Source: CAD feature listing. Evaluate the final solid. Frame: model axes, mm. Face numbers are marked on the shaded views. Round coordinates to 2 decimals unless told otherwise and drop trailing zeros. Loops run counter-clockwise (first coordinate to the right, second up) from the corner with the lowest first, then second, coordinate; pieces in that order, holes last. Notation, with made-up numbers: M 13,88.25 L 68,88.25 A24 cw 68,108.25 Z; hole C 29.5,28.5 d1. An arc over 180 degrees is marked long. One line per item, written item: value.
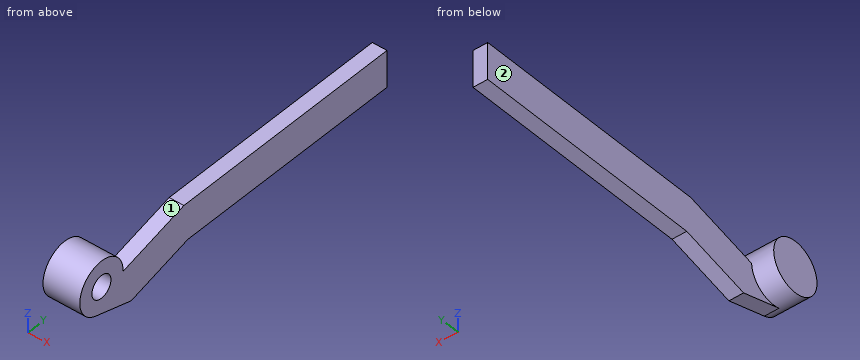
from build123d import *

# Parameters (mm, degrees)
SKETCH1_R           = 7
SKETCH1_R_2         = 3.0845
BOSS_EXTRUDE1_DEPTH = 10
BOSS_EXTRUDE2_START = 7
SKETCH1_3_R         = 7
BOSS_EXTRUDE2_DEPTH = 3
BOSS_EXTRUDE3_DEPTH = 4


with BuildPart() as part:
    # Sketch1 → Boss-Extrude1 (new body)
    with BuildSketch(Plane.ZY.offset(20.145)):
        Circle(SKETCH1_R)
        Circle(SKETCH1_R_2, mode=Mode.SUBTRACT)
    extrude(amount=BOSS_EXTRUDE1_DEPTH)

    # Sketch1<3> → Boss-Extrude2 (add)
    with BuildSketch(Plane.ZY.offset(20.145).offset(BOSS_EXTRUDE2_START)):
        Circle(SKETCH1_3_R)
    extrude(amount=BOSS_EXTRUDE2_DEPTH)

    # Sketch1<5> → Boss-Extrude3 (add)
    with BuildSketch(Plane.ZY.offset(20.145)):
        with BuildLine():
            Line((-5, 92.287872085), (-5, 27.967015644))
            Line((-5, 27.967015644), (-9.925953163, 9.583108165))
            Line((-9.925953163, 9.583108165), (-6.744787083, -1.872924772))
            ThreePointArc((-6.744787083, -1.872924772), (-5.652422268, 4.129179399), (-0.2666949, 6.994917714))
            Line((-0.2666949, 6.994917714), (5, 26.650490668))
            Line((5, 26.650490668), (5, 92.287872085))
            Line((5, 92.287872085), (-5, 92.287872085))
        make_face()
    extrude(amount=BOSS_EXTRUDE3_DEPTH)


solid = part.part
1. Section query A-A (x = -22.75). Return the cut outline in (y, z).
Report:
outline: M -1.87,-6.74 L 9.58,-9.93 L 27.97,-5 L 92.29,-5 L 92.29,5 L 26.65,5 L 6.99,-0.27 A7 ccw long Z; hole C 0,0 d6.17
2. Section query B-B (z = -2). Return the cut outline in (x, y) (3 decimals).
Report:
outline: M -30.145,-6.708 L -20.145,-6.708 L -20.145,-2.348 L -27.145,-2.348 L -27.145,2.348 L -20.145,2.348 L -20.145,92.288 L -24.145,92.288 L -24.145,6.708 L -30.145,6.708 Z
3. Pin query (flat end, axial travel): pin 1 (1.2 mm diameter, centred on x = -22, y = 63.5, fed in from +Z); pin 2 (3 mm diameter, centred on x = -21.5, y = 65.5, fed in from -Z); pin 3 (1 mm diameter, centred on x = -26.5, y = 25, fed in from -Z); pin 4 (4 mm diameter, centred on x = -23, y = 22.5, fed in from +Z). Return the tip coordinate at first contact, or that it passes through.
Report:
pin 1: stops at z = 5
pin 2: stops at z = -5
pin 3: passes through
pin 4: stops at z = 4.42
4. Pull-direction query (Y, two-part tool) for the marked faces 1 and 2; classes: released by +Y, released by -Y, zero draft, split by the parting line, or undercut.
Report:
face 1: undercut
face 2: zero draft
5. Ray query, line 1 (Z direction, x = -24.5, y = 0); line 2 (Z direction, x = -22.25, y = 29.5). Return the intervals inside material, ascending. Write a range as [from, to].
Report:
line 1: z = [-7, -3.08], [3.08, 7]
line 2: z = [-5, 5]
6. Section query D-D (y = 79). Return the cut outline in (x, z) (3 decimals), and give its area (3 significant figures).
Report:
outline: M -24.145,-5 L -20.145,-5 L -20.145,5 L -24.145,5 Z
area: 40.0 mm2
